Geometry check sheet. Reference: the model listing, model coordinates, mm. A direction names the side the tool comes from. Round coordinates to 2 decimals unless told otherwise and drop trailing zeros. Order: outer loops, then holes, each group sorted by start corner. A loop starts at its lowest first (then second) coordinate and runs counter-clockwise, first axis right, second up.
(1) Cross-section at B-B on x = -40.5. Enter the section's corners in (y, z).
(2) Set-up check for faces 1 (the face through (45, 171, -48)), 2 (the face through (-1, 118, -107.5)), 3 (the face through (4, 10, -2)): record each of +Z, -Z, +X, -X, +Y, -Y from which the full face is reachable in a straight line by a thin tool's end or side.
(3) Thickness scan on L1, parallel to Y at x = -14, z = -36.5; L2, parallel to Z at x = 36, y = 81; L3, parallel to X at y = 145, z = 68. Record the ranges inside material, lowest first.
(4) Cross-section at A-A on z = -0.5. Enter the section's corners in (x, y), and give its area (3 significant figures).
(5) Gauge pin test, flat ends, axial feed: P1, Ø10, axis at y = 150.5, z = -52, coming from the +X side; P2, Ø5, axis at x = 13.5, y = 124, coming from the -Z side; P3, Ø12, axis at x = -12, y = 77.5, coming from the +Z side. Record the tip position at first contact, or that the pin passes through.
(6) Cross-section at C-C on y = 191. Enter the section's corners in (x, z), and give its area (3 significant figures).
(7) Cross-section at D-D on x = 6. Enter the section's corners in (y, z), and give its area (3 significant figures).
(8) Draft check along Y on faces 4 (the face through (-3, 110, -9)), 5 (the face through (50, 122, -6)), 6 (the face through (4, 0, -2)). Enter one of: pulls with the +Y half, pulls with the -Y half, needs draft (parallel to the pull), parting line crosses it, or undercut.
from build123d import *

# Parameters (mm, degrees)
SKETCH1_W           = 120
SKETCH1_H           = 235
FLOOR_2_DEPTH       = 10
SKETCH2_W           = 45
SKETCH2_H           = 5
BOSS_EXTRUDE2_DEPTH = 100
SKETCH3_W           = 100
SKETCH3_H           = 200
BOSS_EXTRUDE3_DEPTH = 10
SKETCH4_W           = 45
SKETCH4_H           = 5
BOSS_EXTRUDE4_DEPTH = 100
SKETCH5_W           = 100
SKETCH5_H           = 200
BOSS_EXTRUDE5_DEPTH = 10
SKETCH6_W           = 40
SKETCH6_H           = 15
BOSS_EXTRUDE6_DEPTH = 5
SKETCH7_W           = 90
SKETCH7_H           = 15
BOSS_EXTRUDE7_DEPTH = 5
SKETCH8_W           = 60
SKETCH8_H           = 80
CUT_EXTRUDE1_DEPTH  = 5
SKETCH10_W          = 10
SKETCH10_H          = 235
CUT_EXTRUDE2_DEPTH  = 10


with BuildPart() as part:
    # Sketch1 → floor 2 (new body)
    with BuildSketch(Plane(origin=(0, 0, 0), x_dir=(1, 0, 0), z_dir=(0, 1, 0))):
        Rectangle(SKETCH1_W, SKETCH1_H)
    extrude(amount=FLOOR_2_DEPTH)

    # Sketch2 → Boss-Extrude2 (add)
    with BuildSketch(Plane(origin=(0, 10, 0), x_dir=(1, 0, 0), z_dir=(0, 1, 0))):
        Polygon((-50, 102.5), (-50, 107.5), (50, 107.5), (50, -92.5), (35, -92.5), (35, -87.5), (45, -87.5), (45, 102.5), align=None)
        with Locations((-27.5, -90)):
            Rectangle(SKETCH2_W, SKETCH2_H)
    extrude(amount=BOSS_EXTRUDE2_DEPTH)

    # Sketch3 → Boss-Extrude3 (add)
    with BuildSketch(Plane(origin=(0, 110, 0), x_dir=(1, 0, 0), z_dir=(0, 1, 0))):
        with Locations((0, 7.5)):
            Rectangle(SKETCH3_W, SKETCH3_H)
    extrude(amount=BOSS_EXTRUDE3_DEPTH)

    # Sketch4 → Boss-Extrude4 (add)
    with BuildSketch(Plane(origin=(0, 120, 0), x_dir=(1, 0, 0), z_dir=(0, 1, 0))):
        Polygon((-50, 102.5), (-50, 107.5), (50, 107.5), (50, 42.5), (45, 42.5), (45, 102.5), align=None)
        with Locations((-27.5, -90)):
            Rectangle(SKETCH4_W, SKETCH4_H)
        Polygon((35, -87.5), (35, -92.5), (50, -92.5), (50, -47.5), (45, -47.5), (45, -87.5), align=None)
    extrude(amount=BOSS_EXTRUDE4_DEPTH)

    # Sketch5 → Boss-Extrude5 (add)
    with BuildSketch(Plane(origin=(0, 220, 0), x_dir=(1, 0, 0), z_dir=(0, 1, 0))):
        with Locations((0, 7.5)):
            Rectangle(SKETCH5_W, SKETCH5_H)
    extrude(amount=BOSS_EXTRUDE5_DEPTH)

    # Sketch6 → Boss-Extrude6 (add)
    with BuildSketch(Plane.XY.offset(92.5)):
        with Locations((15, 17.5)):
            Rectangle(SKETCH6_W, SKETCH6_H)
        with Locations((15, 102.5)):
            Rectangle(SKETCH6_W, SKETCH6_H)
        with Locations((15, 127.5)):
            Rectangle(SKETCH6_W, SKETCH6_H)
        with Locations((15, 212.5)):
            Rectangle(SKETCH6_W, SKETCH6_H)
    extrude(amount=-BOSS_EXTRUDE6_DEPTH)

    # Sketch7 → Boss-Extrude7 (add)
    with BuildSketch(Plane(origin=(50, 0, 0), x_dir=(0, 0, -1), z_dir=(1, 0, 0))):
        with Locations((-2.5, 127.5)):
            Rectangle(SKETCH7_W, SKETCH7_H)
        with Locations((-2.5, 212.5)):
            Rectangle(SKETCH7_W, SKETCH7_H)
    extrude(amount=-BOSS_EXTRUDE7_DEPTH)

    # Sketch8 → Cut-Extrude1 (cut)
    with BuildSketch(Plane(origin=(0, 0, -107.5), x_dir=(-1, 0, 0), z_dir=(0, 0, -1))):
        with Locations((0, 50)):
            Rectangle(SKETCH8_W, SKETCH8_H)
        with Locations((0, 160)):
            Rectangle(SKETCH8_W, SKETCH8_H)
    extrude(amount=-CUT_EXTRUDE1_DEPTH, mode=Mode.SUBTRACT)

    # Sketch10 → Cut-Extrude2 (cut)
    with BuildSketch(Plane(origin=(0, 10, 0), x_dir=(1, 0, 0), z_dir=(0, 1, 0))):
        with Locations((-55, 0)):
            Rectangle(SKETCH10_W, SKETCH10_H)
    extrude(amount=-CUT_EXTRUDE2_DEPTH, mode=Mode.SUBTRACT)


solid = part.part
Found:
1. outline: (0, -117.5) - (10, -117.5) - (10, -107.5) - (230, -107.5) - (230, 92.5) - (10, 92.5) - (10, 117.5) - (0, 117.5) - close; hole (10, -102.5) - (110, -102.5) - (110, 87.5) - (10, 87.5) - close; hole (120, -102.5) - (220, -102.5) - (220, 87.5) - (120, 87.5) - close
2. face 1: -X
2. face 2: -Z, +X, -X, +Y
2. face 3: none
3. L1: y = 0 to 10, 110 to 120, 220 to 230
3. L2: z = -107.5 to -102.5, 87.5 to 92.5
3. L3: x = 45 to 50
4. outline: (-50, 0) - (60, 0) - (60, 10) - (50, 10) - (50, 135) - (45, 135) - (45, 120) - (-50, 120) - (-50, 110) - (45, 110) - (45, 10) - (-50, 10) - close; (-50, 220) - (45, 220) - (45, 205) - (50, 205) - (50, 230) - (-50, 230) - close
4. area: 3,750 mm2
5. P1: stops at x = 50
5. P2: stops at z = 87.5
5. P3: stops at z = 92.5
6. outline: (-50, -107.5) - (-30, -107.5) - (-30, -102.5) - (-50, -102.5) - close; (-50, 87.5) - (-5, 87.5) - (-5, 92.5) - (-50, 92.5) - close; (30, -107.5) - (50, -107.5) - (50, -42.5) - (45, -42.5) - (45, -102.5) - (30, -102.5) - close; (35, 87.5) - (45, 87.5) - (45, 47.5) - (50, 47.5) - (50, 92.5) - (35, 92.5) - close
6. area: 1,000 mm2
7. outline: (0, -117.5) - (10, -117.5) - (10, 87.5) - (25, 87.5) - (25, 92.5) - (10, 92.5) - (10, 117.5) - (0, 117.5) - close; (90, -107.5) - (120, -107.5) - (120, 87.5) - (135, 87.5) - (135, 92.5) - (95, 92.5) - (95, 87.5) - (110, 87.5) - (110, -102.5) - (90, -102.5) - close; (200, -107.5) - (230, -107.5) - (230, 92.5) - (205, 92.5) - (205, 87.5) - (220, 87.5) - (220, -102.5) - (200, -102.5) - close
7. area: 6,850 mm2
8. face 4: undercut
8. face 5: needs draft
8. face 6: pulls with the -Y half
